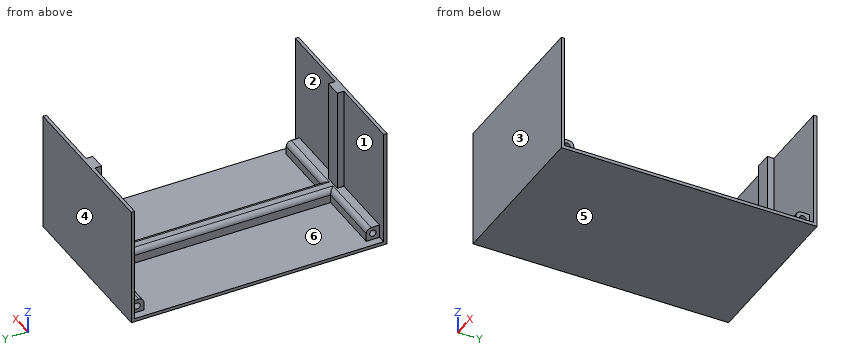
```python
from build123d import *

# Parameters (mm, degrees)
SKETCH1_W           = 154
SKETCH1_H           = 100
BOSS_EXTRUDE1_DEPTH = 2
SKETCH2_W           = 100
SKETCH2_H           = 2
BOSS_EXTRUDE2_DEPTH = 70
SKETCH3_W           = 90.6
SKETCH3_H           = 8
BOSS_EXTRUDE3_DEPTH = 8
SKETCH4_W           = 10
SKETCH4_H           = 134
BOSS_EXTRUDE4_DEPTH = 8
SKETCH5_W           = 10
SKETCH5_H           = 4
BOSS_EXTRUDE5_DEPTH = 62
SKETCH6_R           = 1.95
CUT_EXTRUDE1_DEPTH  = 195.889943301
SKETCH7_R           = 1.95
CUT_EXTRUDE2_DEPTH  = 195.889943301
FILLET1_R           = 3


with BuildPart() as part:
    # Sketch1 → Boss-Extrude1 (new body)
    with BuildSketch(Plane(origin=(0, 0, 0), x_dir=(0, 1, 0), z_dir=(0, 0, 1))):
        with Locations((77, 50)):
            Rectangle(SKETCH1_W, SKETCH1_H)
    extrude(amount=BOSS_EXTRUDE1_DEPTH)

    # Sketch2 → Boss-Extrude2 (add)
    with BuildSketch(Plane.XY.offset(2)):
        with Locations((-50, 153)):
            Rectangle(SKETCH2_W, SKETCH2_H)
        with Locations((-50, 1)):
            Rectangle(SKETCH2_W, SKETCH2_H)
    extrude(amount=BOSS_EXTRUDE2_DEPTH)

    # Sketch3 → Boss-Extrude3 (add)
    with BuildSketch(Plane.XY.offset(2)):
        with Locations((-50, 148)):
            Rectangle(SKETCH3_W, SKETCH3_H)
        with Locations((-50, 6)):
            Rectangle(SKETCH3_W, SKETCH3_H)
    extrude(amount=BOSS_EXTRUDE3_DEPTH)

    # Sketch4 → Boss-Extrude4 (add)
    with BuildSketch(Plane.XY.offset(2)):
        with Locations((-50, 77)):
            Rectangle(SKETCH4_W, SKETCH4_H)
    extrude(amount=BOSS_EXTRUDE4_DEPTH)

    # Sketch5 → Boss-Extrude5 (add)
    with BuildSketch(Plane.XY.offset(10)):
        with Locations((-50, 150)):
            Rectangle(SKETCH5_W, SKETCH5_H)
        with Locations((-50, 4)):
            Rectangle(SKETCH5_W, SKETCH5_H)
    extrude(amount=BOSS_EXTRUDE5_DEPTH)

    # Sketch6 → Cut-Extrude1 (cut, through all)
    with BuildSketch(Plane(origin=(-95.3, 0, 0), x_dir=(0, -1, 0), z_dir=(-1, 0, 0))):
        with Locations((-6, 6)):
            Circle(SKETCH6_R)
    extrude(amount=-CUT_EXTRUDE1_DEPTH, mode=Mode.SUBTRACT)

    # Sketch7 → Cut-Extrude2 (cut, through all)
    with BuildSketch(Plane(origin=(-95.3, 0, 0), x_dir=(0, -1, 0), z_dir=(-1, 0, 0))):
        with Locations(Location((-148, 6, 0), (0, 0, 90))):
            Circle(SKETCH7_R)
    extrude(amount=-CUT_EXTRUDE2_DEPTH, mode=Mode.SUBTRACT)

    # Fillet1
    fillet1_edges = [part.edges().sort_by_distance(p)[0] for p in [
        (-75.15, 144, 10),
        (-24.85, 10, 10),
        (-75.15, 10, 10),
        (-24.85, 144, 10),
        (-55, 77, 10),
        (-45, 77, 10),
    ]]
    fillet(fillet1_edges, radius=FILLET1_R)


solid = part.part
```
Part model, mm, in its own coordinate system. Face numbers are marked on the shaded views. A direction names the side the tool comes from. Coordinates: 2 decimals unless noted, no trailing zeros. Write each loop counter-clockwise with the first axis right and the second up, starting at its lowest first coordinate (ties: lowest second). Pieces come first, ordered by that corner, then holes.
Item 1: Pin check, flat tips, straight feed: pin 1 (8 mm diameter, centred on x = -16.5, y = 29, fed in from +Z); pin 2 (1.2 mm diameter, centred on y = 149.5, z = 37.5, fed in from +X); pin 3 (4.5 mm diameter, centred on y = 148, z = 6, fed in from -X). Stop position of each tip, or through.
Item 2: Mould opens along Y. For the marked faces 3, 4, 5 and 6 say: released by +Y, released by -Y, zero draft, split by the parting line, or undercut.
Item 3: Slice it at A-A (z = 33.5). Write the cut outline in (x, y), and give its area (3 significant figures).
Item 4: Slice it at B-B (x = -91). Write the cut outline in (y, z).
Item 5: Probe line 1 (Y direction, x = -53, z = 35); line 2 (Y direction, x = -83, z = 44); line 3 (Z direction, x = -74, y = 6). List the from-to ranges inside material, lowest first.
Item 6: Slice it at C-C (y = 45). Write the cut outline in (x, z).
Item 7: Which spindle directions (+Z, -Z, +X, -X, +Y, -Y) get a long thin tool onto all of the face, cutting with end or side? Do the marked faces 1 and 2. Say none if no direction does.
Results found:
1. pin 1: stops at z = 2
1. pin 2: stops at x = -45
1. pin 3: stops at x = -95.3
2. face 3: released by -Y
2. face 4: released by +Y
2. face 5: zero draft
2. face 6: undercut
3. outline: (-100, 0) - (0, 0) - (0, 2) - (-45, 2) - (-45, 6) - (-55, 6) - (-55, 2) - (-100, 2) - close; (-100, 152) - (-55, 152) - (-55, 148) - (-45, 148) - (-45, 152) - (0, 152) - (0, 154) - (-100, 154) - close
3. area: 480 mm2
4. outline: (0, 0) - (154, 0) - (154, 72) - (152, 72) - (152, 10) - (147, 10) arc R3 ccw to (144, 7) - (144, 2) - (10, 2) - (10, 7) arc R3 ccw to (7, 10) - (2, 10) - (2, 72) - (0, 72) - close; hole circle Ø3.9 at (6, 6); hole circle Ø3.9 at (148, 6)
5. line 1: y = 0 to 6, 148 to 154
5. line 2: y = 0 to 2, 152 to 154
5. line 3: z = 0 to 4.05, 7.95 to 10
6. outline: (-100, 0) - (0, 0) - (0, 2) - (-45, 2) - (-45, 7) arc R3 ccw to (-48, 10) - (-52, 10) arc R3 ccw to (-55, 7) - (-55, 2) - (-100, 2) - close
7. face 1: +Z, -X
7. face 2: +Z, +X
